from build123d import *

# Parameters (mm, degrees)
CROQUIS1_W              = 250
CROQUIS1_H              = 250
CROQUIS1_R              = 2.5
SALIENTE_EXTRUIR1_DEPTH = 4
CORTAR_EXTRUIR1_DEPTH   = 4
CROQUIS3_W              = 150
CROQUIS3_H              = 150
CROQUIS3_W_2            = 100
CROQUIS3_H_2            = 100
SALIENTE_EXTRUIR2_DEPTH = 4
CROQUIS4_R              = 1.55
CORTAR_EXTRUIR2_DEPTH   = 10
CROQUIS5_W              = 150
CROQUIS5_H              = 150
CROQUIS5_W_2            = 100
CROQUIS5_H_2            = 100
CORTAR_EXTRUIR3_DEPTH   = 10
CROQUIS6_R              = 1.55
CORTAR_EXTRUIR4_DEPTH   = 10


with BuildPart() as part:
    # Croquis1 → Saliente-Extruir1 (new body)
    with BuildSketch(Plane(origin=(0, 0, 0), x_dir=(1, 0, 0), z_dir=(0, 1, 0))):
        with Locations((125, 125)):
            Rectangle(CROQUIS1_W, CROQUIS1_H)
        with Locations(Location((40, 210, 0), (0, 0, 270))):
            Circle(CROQUIS1_R, mode=Mode.SUBTRACT)
        with Locations(Location((210, 210, 0), (0, 0, 270))):
            Circle(CROQUIS1_R, mode=Mode.SUBTRACT)
        with Locations(Location((210, 40, 0), (0, 0, 270))):
            Circle(CROQUIS1_R, mode=Mode.SUBTRACT)
        with Locations(Location((40, 40, 0), (0, 0, 270))):
            Circle(CROQUIS1_R, mode=Mode.SUBTRACT)
    extrude(amount=SALIENTE_EXTRUIR1_DEPTH)

    # Croquis2 → Cortar-Extruir1 (cut)
    with BuildSketch(Plane(origin=(0, 4, 0), x_dir=(1, 0, 0), z_dir=(0, 1, 0))):
        Polygon((50, 50), (200, 50), (200, 200), (50, 200), (50, 150.09044268), align=None)
    extrude(amount=-CORTAR_EXTRUIR1_DEPTH, mode=Mode.SUBTRACT)

    # Croquis3 → Saliente-Extruir2 (add)
    with BuildSketch(Plane(origin=(0, 4, 0), x_dir=(1, 0, 0), z_dir=(0, 1, 0))):
        with Locations((125, 125)):
            Rectangle(CROQUIS3_W, CROQUIS3_H)
        with Locations((125, 125)):
            Rectangle(CROQUIS3_W_2, CROQUIS3_H_2, mode=Mode.SUBTRACT)
    extrude(amount=-SALIENTE_EXTRUIR2_DEPTH)

    # Croquis4 → Cortar-Extruir2 (cut)
    with BuildSketch(Plane(origin=(0, 4, 0), x_dir=(1, 0, 0), z_dir=(0, 1, 0))):
        with Locations(Location((115, 20, 0), (0, 0, 270))):
            Circle(CROQUIS4_R)
        with Locations(Location((135, 20, 0), (0, 0, 270))):
            Circle(CROQUIS4_R)
        with Locations(Location((125, 5, 0), (0, 0, 270))):
            Circle(CROQUIS4_R)
    extrude(amount=-CORTAR_EXTRUIR2_DEPTH, mode=Mode.SUBTRACT)

    # Croquis5 → Cortar-Extruir3 (cut)
    with BuildSketch(Plane(origin=(0, 4, 0), x_dir=(1, 0, 0), z_dir=(0, 1, 0))):
        with Locations((125, 125)):
            Rectangle(CROQUIS5_W, CROQUIS5_H)
        with Locations((125, 125)):
            Rectangle(CROQUIS5_W_2, CROQUIS5_H_2, mode=Mode.SUBTRACT)
    extrude(amount=-CORTAR_EXTRUIR3_DEPTH, mode=Mode.SUBTRACT)

    # Croquis6 → Cortar-Extruir4 (cut)
    with BuildSketch(Plane(origin=(0, 4, 0), x_dir=(1, 0, 0), z_dir=(0, 1, 0))):
        with Locations(Location((125, 5, 0), (0, 0, 270))):
            Circle(CROQUIS6_R)
        with Locations(Location((115, 20, 0), (0, 0, 270))):
            Circle(CROQUIS6_R)
        with Locations(Location((135, 20, 0), (0, 0, 270))):
            Circle(CROQUIS6_R)
        with Locations(Location((20, 115, 0), (0, 0, 270))):
            Circle(CROQUIS6_R)
        with Locations(Location((20, 135, 0), (0, 0, 270))):
            Circle(CROQUIS6_R)
        with Locations(Location((5, 125, 0), (0, 0, 270))):
            Circle(CROQUIS6_R)
        with Locations(Location((115, 230, 0), (0, 0, 270))):
            Circle(CROQUIS6_R)
        with Locations(Location((135, 230, 0), (0, 0, 270))):
            Circle(CROQUIS6_R)
        with Locations(Location((125, 245, 0), (0, 0, 270))):
            Circle(CROQUIS6_R)
        with Locations(Location((230, 135, 0), (0, 0, 270))):
            Circle(CROQUIS6_R)
        with Locations(Location((230, 115, 0), (0, 0, 270))):
            Circle(CROQUIS6_R)
        with Locations(Location((245, 125, 0), (0, 0, 270))):
            Circle(CROQUIS6_R)
    extrude(amount=-CORTAR_EXTRUIR4_DEPTH, mode=Mode.SUBTRACT)


solid = part.part
Source: CAD feature listing. Evaluate the final solid. Frame: model axes, mm. Round coordinates to 2 decimals unless told otherwise and drop trailing zeros. Loops run counter-clockwise (first coordinate to the right, second up) from the corner with the lowest first, then second, coordinate; pieces in that order, holes last.
Q1. First-contact query: P1, Ø2.5, axis at x = 135, z = -230, coming from the -Y side. Flat tip, straight axial feed; report the tip coordinate or a pass-through.
Q2. Ray query, line 1 (X direction, y = 2.7, z = -115); line 2 (X direction, y = 2.05, z = -230); line 3 (Z direction, x = 135, y = 1.65). Return the intervals inside material, ascending.
Q3. Section B-B, the plane y = 0.95. State how many separate pieces and enclosed holes the cut face has, plus the area to 3 significant figures.
Q4. Section C-C, the plane z = -83. Return loops of the section in (x, y).
Q5. Section A-A, the plane x = 83. Return loops of the section in (y, z), plus the area to 3 significant figures.
Solutions:
1. P1: passes through
2. line 1: x = 0 to 18.45, 21.55 to 50, 200 to 228.45, 231.55 to 250
2. line 2: x = 0 to 113.45, 116.55 to 133.45, 136.55 to 250
2. line 3: z = -250 to -231.55, -228.45 to -200, -50 to -21.55, -18.45 to 0
3. separate pieces: 1
3. enclosed holes: 17
3. area: 39,800 mm2
4. outline: (0, 0) - (50, 0) - (50, 4) - (0, 4) - close; (200, 0) - (250, 0) - (250, 4) - (200, 4) - close
5. outline: (0, -250) - (4, -250) - (4, -200) - (0, -200) - close; (0, -50) - (4, -50) - (4, 0) - (0, 0) - close
5. area: 400 mm2
